Here's how the part is built. I have some questions about the finished solid (model axes, mm). A direction names the side the tool comes from. Coordinates: 2 decimals unless noted, no trailing zeros. Write each loop counter-clockwise with the first axis right and the second up, starting at its lowest first coordinate (ties: lowest second). Pieces come first, ordered by that corner, then holes.
Item 1: For faces 1 (the face through (19.647, -53.467, 1.109)), 2 (the face through (-18, -29, 1)), 3 (the face through (-5.18, -9.73, 1.11)), which set-ups out of +Z, -Z, +X, -X, +Y, -Y let a thin tool reach every point of the face, with its end or its side?
Item 2: I want a section at A-A (y = -28.25). Please give me the cut outline in (x, z).
Item 3: I'm going to push a flat-ended pin straight in: P1, Ø3.5, axis at x = 16.5, y = -28.25, coming from the +Z side. Where does the tip first touch, or does it pass through?
Item 4: If we mould it in two halves opening along Y, with no side actions, what happens to faces 4 (the face through (-19.717, -53.397, 1.109)), 5 (the face through (-5.32, 29.23, 1.11)), 6 (the face through (0, 39.75, 1))? For each: pulls with the +Y half, pulls with the -Y half, needs draft (parallel to the pull), parting line crosses it, or undercut.
Item 5: I want a section at D-D (y = 32.25). Please give me the cut outline in (x, z), and give its area (3 significant figures).
Item 6: Please list where these lines run through material, in increasing order: line 1 (Y direction, x = 16.5, z = 0.6); line 2 (Y direction, x = 16.5, z = 1.65).
Item 7: I want a section at C-C (y = -7). Please give me the cut outline in (x, z) (3 decimals), and give its area (3 significant figures).
Item 8: I want a section at B-B (y = 17.5). Please give me the cut outline in (x, z) (3 decimals), and give its area (3 significant figures).
from build123d import *

# Parameters (mm, degrees)
F0_R     = 1.5
F1_DEPTH = 2.25
F2_R     = 3
F3_DEPTH = 1.25


with BuildPart() as f1:
    # F0 (on Top) → F1 (new body)
    with BuildSketch(Plane.XY):
        with BuildLine():
            ThreePointArc((-16.5, 39.75), (-19.681981, 38.431981), (-21, 35.25))
            Line((-21, 35.25), (-21, -44.25))
            Line((-21, -44.25), (-21, -50.25))
            ThreePointArc((-21, -50.25), (-19.681981, -53.431981), (-16.5, -54.75))
            Line((-16.5, -54.75), (16.5, -54.75))
            ThreePointArc((16.5, -54.75), (19.681981, -53.431981), (21, -50.25))
            Line((21, -50.25), (21, -44.25))
            Line((21, -44.25), (21, 35.25))
            ThreePointArc((21, 35.25), (19.681981, 38.431981), (16.5, 39.75))
            Line((16.5, 39.75), (-16.5, 39.75))
        make_face()
        with Locations((-16.5, -28.25)):
            Circle(F0_R, mode=Mode.SUBTRACT)
        with BuildLine():
            ThreePointArc((-16.5, -0.25), (-15.43934, -0.68934), (-15, -1.75))
            Line((-15, -1.75), (-15, -22.25))
            ThreePointArc((-15, -22.25), (-15.43934, -23.31066), (-16.5, -23.75))
            ThreePointArc((-16.5, -23.75), (-17.56066, -23.31066), (-18, -22.25))
            Line((-18, -22.25), (-18, -1.75))
            ThreePointArc((-18, -1.75), (-17.56066, -0.68934), (-16.5, -0.25))
        make_face(mode=Mode.SUBTRACT)
        Polygon((-10.5, -44.25), (0, -41.25), (10.5, -44.25), (10.5, -47.25), (0, -44.25), (-10.5, -47.25), align=None, mode=Mode.SUBTRACT)
        Polygon((-10.5, -38.25), (0, -35.25), (10.5, -38.25), (10.5, -41.25), (0, -38.25), (-10.5, -41.25), align=None, mode=Mode.SUBTRACT)
        Polygon((-10.5, -32.25), (0, -29.25), (10.5, -32.25), (10.5, -35.25), (0, -32.25), (-10.5, -35.25), align=None, mode=Mode.SUBTRACT)
        Polygon((-10.5, -26.25), (0, -23.25), (10.5, -26.25), (10.5, -29.25), (0, -26.25), (-10.5, -29.25), align=None, mode=Mode.SUBTRACT)
        Polygon((-10.5, -20.25), (0, -17.25), (10.5, -20.25), (10.5, -23.25), (0, -20.25), (-10.5, -23.25), align=None, mode=Mode.SUBTRACT)
        Polygon((-10.5, -14.25), (0, -11.25), (10.5, -14.25), (10.5, -17.25), (0, -14.25), (-10.5, -17.25), align=None, mode=Mode.SUBTRACT)
        Polygon((-10.5, -8.25), (0, -5.25), (10.5, -8.25), (10.5, -11.25), (0, -8.25), (-10.5, -11.25), align=None, mode=Mode.SUBTRACT)
        with Locations((16.5, -28.25)):
            Circle(F0_R, mode=Mode.SUBTRACT)
        with BuildLine():
            ThreePointArc((16.5, -0.25), (17.56066, -0.68934), (18, -1.75))
            Line((18, -1.75), (18, -22.25))
            ThreePointArc((18, -22.25), (17.56066, -23.31066), (16.5, -23.75))
            ThreePointArc((16.5, -23.75), (15.43934, -23.31066), (15, -22.25))
            Line((15, -22.25), (15, -1.75))
            ThreePointArc((15, -1.75), (15.43934, -0.68934), (16.5, -0.25))
        make_face(mode=Mode.SUBTRACT)
        with Locations((-16.5, 32.25)):
            Circle(F0_R, mode=Mode.SUBTRACT)
        Polygon((-10.5, -2.25), (0, 0.75), (10.5, -2.25), (10.5, -5.25), (0, -2.25), (-10.5, -5.25), align=None, mode=Mode.SUBTRACT)
        Polygon((-10.5, 3.75), (0, 6.75), (10.5, 3.75), (10.5, 0.75), (0, 3.75), (-10.5, 0.75), align=None, mode=Mode.SUBTRACT)
        Polygon((-10.5, 9.75), (0, 12.75), (10.5, 9.75), (10.5, 6.75), (0, 9.75), (-10.5, 6.75), align=None, mode=Mode.SUBTRACT)
        Polygon((-10.5, 15.75), (0, 18.75), (10.5, 15.75), (10.5, 12.75), (0, 15.75), (-10.5, 12.75), align=None, mode=Mode.SUBTRACT)
        Polygon((-10.5, 21.75), (0, 24.75), (10.5, 21.75), (10.5, 18.75), (0, 21.75), (-10.5, 18.75), align=None, mode=Mode.SUBTRACT)
        Polygon((-10.5, 27.75), (0, 30.75), (10.5, 27.75), (10.5, 24.75), (0, 27.75), (-10.5, 24.75), align=None, mode=Mode.SUBTRACT)
        Polygon((-10.5, 33.75), (0, 36.75), (10.5, 33.75), (10.5, 30.75), (0, 33.75), (-10.5, 30.75), align=None, mode=Mode.SUBTRACT)
        with Locations((16.5, 32.25)):
            Circle(F0_R, mode=Mode.SUBTRACT)
    extrude(amount=F1_DEPTH)

    # F2 (on face) → F3 (cut)
    with BuildSketch(Plane.XY.offset(2.25)):
        with Locations((-16.5, -28.25)):
            Circle(F2_R)
        with Locations((16.5, -28.25)):
            Circle(F2_R)
        with Locations((16.5, 32.25)):
            Circle(F2_R)
        with Locations((-16.5, 32.25)):
            Circle(F2_R)
    extrude(amount=-F3_DEPTH, mode=Mode.SUBTRACT)


solid = f1.part
Answer:
1. face 1: +Z, -Z, +X, -Y
1. face 2: +Z
1. face 3: +Z, -Z
2. outline: (-21, 0) - (-18, 0) - (-18, 1) - (-19.5, 1) - (-19.5, 2.25) - (-21, 2.25) - close; (-15, 0) - (-10.5, 0) - (-10.5, 2.25) - (-13.5, 2.25) - (-13.5, 1) - (-15, 1) - close; (-7, 0) - (7, 0) - (7, 2.25) - (-7, 2.25) - close; (10.5, 0) - (15, 0) - (15, 1) - (13.5, 1) - (13.5, 2.25) - (10.5, 2.25) - close; (18, 0) - (21, 0) - (21, 2.25) - (19.5, 2.25) - (19.5, 1) - (18, 1) - close
3. P1: stops at z = 1
4. face 4: pulls with the -Y half
4. face 5: undercut
4. face 6: pulls with the +Y half
5. outline: (-21, 0) - (-18, 0) - (-18, 1) - (-19.5, 1) - (-19.5, 2.25) - (-21, 2.25) - close; (-15, 0) - (-10.5, 0) - (-10.5, 2.25) - (-13.5, 2.25) - (-13.5, 1) - (-15, 1) - close; (-5.25, 0) - (5.25, 0) - (5.25, 2.25) - (-5.25, 2.25) - close; (10.5, 0) - (15, 0) - (15, 1) - (13.5, 1) - (13.5, 2.25) - (10.5, 2.25) - close; (18, 0) - (21, 0) - (21, 2.25) - (19.5, 2.25) - (19.5, 1) - (18, 1) - close
5. area: 49.9 mm2
6. line 1: y = -54.75 to -29.75, -26.75 to -23.75, -0.25 to 30.75, 33.75 to 39.75
6. line 2: y = -54.75 to -31.25, -25.25 to -23.75, -0.25 to 29.25, 35.25 to 39.75
7. outline: (-21, 0) - (-18, 0) - (-18, 2.25) - (-21, 2.25) - close; (-15, 0) - (-6.125, 0) - (-6.125, 2.25) - (-15, 2.25) - close; (6.125, 0) - (15, 0) - (15, 2.25) - (6.125, 2.25) - close; (18, 0) - (21, 0) - (21, 2.25) - (18, 2.25) - close
7. area: 53.4 mm2
8. outline: (-21, 0) - (-4.375, 0) - (-4.375, 2.25) - (-21, 2.25) - close; (4.375, 0) - (21, 0) - (21, 2.25) - (4.375, 2.25) - close
8. area: 74.8 mm2
